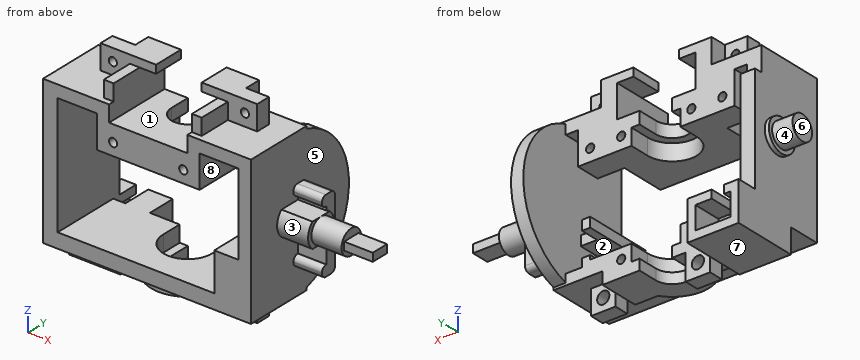
```python
from build123d import *

# Parameters (mm, degrees)
SKETCH_1_R               = 0.5
EXTRUDE_1_DEPTH          = 8.5
SKETCH_2_W               = 3.3
SKETCH_2_H               = 4
SKETCH_2_R               = 0.5
EXTRUDE_2_DEPTH          = 3
EXTRUDE_3_DEPTH          = 3.8
SKETCH_4_W               = 2.8
SKETCH_4_H               = 3
SKETCH_4_R               = 0.5
EXTRUDE_4_DEPTH          = 1.8
SKETCH_5_W               = 1.2
SKETCH_5_H               = 2
EXTRUDE_5_DEPTH          = 4
SKETCH_6_W               = 1.8
SKETCH_6_H               = 15
EXTRUDE_6_DEPTH          = 1
EXTRUDE_7_DEPTH          = 3.5
EXTRUDE_7_DEPTH_BACK     = 4.5
SKETCH_8_W               = 4.3
SKETCH_8_H               = 2
EXTRUDE_8_DEPTH          = 1
EXTRUDE_9_DEPTH          = 1.5
SKETCH_10_R              = 0.75
EXTRUDE_10_DEPTH         = 1.8
SKETCH_12_W              = 3
SKETCH_12_H              = 1.8
EXTRUDE_11_DEPTH         = 3
SKETCH_13_R              = 0.75
CUT_EXTRUDE_1_DEPTH      = 3
SKETCH_14_R              = 0.5
CUT_EXTRUDE_2_DEPTH      = 3
CUT_EXTRUDE_3_DEPTH      = 7
CUT_EXTRUDE_4_DEPTH      = 36.146123542
CUT_EXTRUDE_5_DEPTH      = 12.7
CUT_EXTRUDE_5_DEPTH_BACK = 2
SKETCH_18_W              = 2
SKETCH_18_H              = 1.2
CUT_EXTRUDE_6_DEPTH      = 2.3
EXTRUDE_12_DEPTH         = 1.5
SKETCH_22_R              = 1.5
EXTRUDE_13_DEPTH         = 3
SKETCH_23_R              = 2
EXTRUDE_14_DEPTH         = 0.5
EXTRUDE_START            = 7.5
SKETCH_24_R              = 1.5
EXTRUDE_15_DEPTH         = 7.5
EXTRUDE_16_DEPTH         = 3.5
EXTRUDE_17_DEPTH         = 3.5
EXTRUDE_START_2          = 3.8
EXTRUDE_18_DEPTH         = 3.8


with BuildPart() as part:
    # 草图1 → 凸台-拉伸1 (new body)
    with BuildSketch(Plane(origin=(0, 0, 0), x_dir=(1, 0, 0), z_dir=(0, 1, 0))):
        Polygon((25.5, 0), (25.5, 18), (0, 18), (0, 0), (8.1, 0), (8.1, 2), (17.7, 2), (17.7, 0), align=None)
        with Locations(Location((8.6, 4, 0), (0, 0, 270))):
            Circle(SKETCH_1_R, mode=Mode.SUBTRACT)
        with Locations(Location((17.2, 4, 0), (0, 0, 270))):
            Circle(SKETCH_1_R, mode=Mode.SUBTRACT)
        Polygon((24, 1.5), (19.2, 1.5), (19.2, 5.5), (12.9, 5.5), (6.6, 5.5), (6.6, 1.5), (1.8, 1.5), (1.8, 16.2), (21, 16.2), (21, 11.5), (24, 11.5), align=None, mode=Mode.SUBTRACT)
    extrude(amount=EXTRUDE_1_DEPTH)

    # 草图2 → 凸台-拉伸2 (add)
    # profile 1 of 2: a face of its own
    with BuildSketch(Plane(origin=(0, 8.5, 0), x_dir=(1, 0, 0), z_dir=(0, 1, 0))):
        with Locations((4.95, 3.5)):
            Rectangle(SKETCH_2_W, SKETCH_2_H)
        with Locations(Location((4.8, 4, 0), (0, 0, 270))):
            Circle(SKETCH_2_R, mode=Mode.SUBTRACT)
    # profile 2 of 2: a face of its own
    with BuildSketch(Plane(origin=(0, 8.5, 0), x_dir=(1, 0, 0), z_dir=(0, 1, 0))):
        with Locations((20.85, 3.5)):
            Rectangle(SKETCH_2_W, SKETCH_2_H)
        with Locations(Location((21, 4, 0), (0, 0, 270))):
            Circle(SKETCH_2_R, mode=Mode.SUBTRACT)
    extrude(amount=-EXTRUDE_2_DEPTH)

    # 草图3 → 凸台-拉伸3 (add)
    with BuildSketch(Plane(origin=(0, 8.5, 0), x_dir=(1, 0, 0), z_dir=(0, 1, 0))):
        Polygon((17.7, 0), (17.7, -2), (15.7, -2), (15.7, -3), (17.7, -3), (19.7, -3), (19.7, 0), align=None)
        Polygon((8.1, 0), (6.1, 0), (6.1, -3), (8.1, -3), (10.1, -3), (10.1, -2), (8.1, -2), align=None)
    extrude(amount=-EXTRUDE_3_DEPTH)

    # 草图4 → 凸台-拉伸4 (add)
    # profile 1 of 2: a face of its own
    with BuildSketch(Plane.XZ.offset(-4.7)):
        with Locations((21.1, 1.5)):
            Rectangle(SKETCH_4_W, SKETCH_4_H)
        with Locations(Location((21, 1.5, 0), (0, 0, 270))):
            Circle(SKETCH_4_R, mode=Mode.SUBTRACT)
    # profile 2 of 2: a face of its own
    with BuildSketch(Plane.XZ.offset(-4.7)):
        with Locations((4.7, 1.5)):
            Rectangle(SKETCH_4_W, SKETCH_4_H)
        with Locations(Location((4.8, 1.5, 0), (0, 0, 270))):
            Circle(SKETCH_4_R, mode=Mode.SUBTRACT)
    extrude(amount=-EXTRUDE_4_DEPTH)

    # 草图5 → 凸台-拉伸5 (add)
    with BuildSketch(Plane.XZ.offset(-4.7)):
        with Locations((7.5, 1)):
            Rectangle(SKETCH_5_W, SKETCH_5_H)
        with Locations((18.3, 1)):
            Rectangle(SKETCH_5_W, SKETCH_5_H)
    extrude(amount=EXTRUDE_5_DEPTH)

    # 草图6 → 凸台-拉伸6 (add)
    with BuildSketch(Plane(origin=(0, 8.5, 0), x_dir=(1, 0, 0), z_dir=(0, 1, 0))):
        with Locations((0.9, 10.5)):
            Rectangle(SKETCH_6_W, SKETCH_6_H)
    extrude(amount=EXTRUDE_6_DEPTH)

    # 草图7 → 凸台-拉伸7 (add, two sides: drawn at the far end of the back side and taken through both)
    with BuildSketch(Plane(origin=(0, 8.5, 0), x_dir=(1, 0, 0), z_dir=(0, 1, 0)).offset(-EXTRUDE_7_DEPTH_BACK)):
        Polygon((0, 18), (0, 21), (6.3, 21), (6.3, 16.2), (3.3, 16.2), (3.3, 17.2), (5.3, 17.2), (5.3, 20), (1, 20), (1, 17.2), (1.8, 17.2), (1.8, 16.2), (0, 16.2), align=None)
    extrude(amount=EXTRUDE_7_DEPTH + EXTRUDE_7_DEPTH_BACK)

    # 草图8 → 凸台-拉伸8 (add)
    with BuildSketch(Plane.XZ.offset(-4)):
        with Locations((3.15, -19)):
            Rectangle(SKETCH_8_W, SKETCH_8_H)
    extrude(amount=-EXTRUDE_8_DEPTH)

    # 草图9 → 凸台-拉伸9 (add)
    with BuildSketch(Plane(origin=(0, 0, -18), x_dir=(-1, 0, 0), z_dir=(0, 0, -1))):
        with BuildLine():
            Line((-10.95, 8.5), (-10.95, 6))
            ThreePointArc((-10.95, 6), (-12.95, 4), (-14.95, 6))
            Line((-14.95, 6), (-14.95, 8.5))
            Line((-14.95, 8.5), (-19.5, 8.5))
            Line((-19.5, 8.5), (-19.5, 3.5))
            Line((-19.5, 3.5), (-16.691657387, 3.5))
            ThreePointArc((-16.691657387, 3.5), (-12.95, 1.5), (-9.208342613, 3.5))
            Line((-9.208342613, 3.5), (-6.3, 3.5))
            Line((-6.3, 3.5), (-6.3, 8.5))
            Line((-6.3, 8.5), (-10.95, 8.5))
        make_face()
    extrude(amount=EXTRUDE_9_DEPTH)

    # 草图10 → 凸台-拉伸10 (add)
    with BuildSketch(Plane(origin=(0, 8.5, 0), x_dir=(1, 0, 0), z_dir=(0, 1, 0))):
        Polygon((6.3, 22.7), (6.3, 19.5), (9.3, 19.5), (9.3, 21.1), (9.3, 22.7), align=None)
        with Locations(Location((7.8, 21.1, 0), (0, 0, 270))):
            Circle(SKETCH_10_R, mode=Mode.SUBTRACT)
    extrude(amount=-EXTRUDE_10_DEPTH)

    # 草图12 → 凸台-拉伸11 (add)
    with BuildSketch(Plane(origin=(0, 0, -18), x_dir=(-1, 0, 0), z_dir=(0, 0, -1))):
        with Locations((-21, 5.6)):
            Rectangle(SKETCH_12_W, SKETCH_12_H)
    extrude(amount=EXTRUDE_11_DEPTH)

    # 草图13 → 切除-拉伸1 (cut)
    with BuildSketch(Plane(origin=(0, 6.5, 0), x_dir=(1, 0, 0), z_dir=(0, 1, 0))):
        with Locations(Location((21, 19.5, 0), (0, 0, 270))):
            Circle(SKETCH_13_R)
    extrude(amount=-CUT_EXTRUDE_1_DEPTH, mode=Mode.SUBTRACT)

    # 草图14 → 切除-拉伸2 (cut)
    with BuildSketch(Plane(origin=(0, 8.5, 0), x_dir=(1, 0, 0), z_dir=(0, 1, 0))):
        with Locations(Location((17.2, 17.5, 0), (0, 0, 270))):
            Circle(SKETCH_14_R)
        with Locations(Location((8.6, 17.5, 0), (0, 0, 270))):
            Circle(SKETCH_14_R)
    extrude(amount=-CUT_EXTRUDE_2_DEPTH, mode=Mode.SUBTRACT)

    # 草图15 → 切除-拉伸3 (cut)
    with BuildSketch(Plane(origin=(0, 8.5, 0), x_dir=(1, 0, 0), z_dir=(0, 1, 0))):
        Polygon((21, 15.7), (21, 12.7), (24, 12.7), (24, 16.7), (22, 16.7), (22, 15.7), align=None)
    extrude(amount=-CUT_EXTRUDE_3_DEPTH, mode=Mode.SUBTRACT)

    # 草图16 → 切除-拉伸4 (cut, through all)
    with BuildSketch(Plane(origin=(0, 0, -18), x_dir=(-1, 0, 0), z_dir=(0, 0, -1))):
        with BuildLine():
            Line((-14.95, 8.5), (-10.95, 8.5))
            Line((-10.95, 8.5), (-10.95, 6))
            ThreePointArc((-10.95, 6), (-12.95, 4), (-14.95, 6))
            Line((-14.95, 6), (-14.95, 8.5))
        make_face()
    extrude(amount=-CUT_EXTRUDE_4_DEPTH, mode=Mode.SUBTRACT)

    # 草图17 → 切除-拉伸5 (cut, two sides: drawn at the far end of the back side and taken through both)
    with BuildSketch(Plane.XY.offset(-16.2).offset(-CUT_EXTRUDE_5_DEPTH_BACK)):
        with BuildLine():
            Line((15.95, 6), (15.95, 8.5))
            Line((15.95, 8.5), (9.95, 8.5))
            Line((9.95, 8.5), (9.95, 6))
            ThreePointArc((9.95, 6), (12.95, 3), (15.95, 6))
        make_face()
    extrude(amount=CUT_EXTRUDE_5_DEPTH + CUT_EXTRUDE_5_DEPTH_BACK, mode=Mode.SUBTRACT)

    # 草图18 → 切除-拉伸6 (cut)
    with BuildSketch(Plane(origin=(0, 8.5, 0), x_dir=(1, 0, 0), z_dir=(0, 1, 0))):
        with Locations((23, 12.1)):
            Rectangle(SKETCH_18_W, SKETCH_18_H)
    extrude(amount=-CUT_EXTRUDE_6_DEPTH, mode=Mode.SUBTRACT)

    # 草图19 → 凸台-拉伸12 (add)
    with BuildSketch(Plane(origin=(25.5, 0, 0), x_dir=(0, 0, -1), z_dir=(1, 0, 0))):
        with BuildLine():
            Line((0.30001254, 8.5), (17.69998746, 8.5))
            ThreePointArc((17.69998746, 8.5), (9, 14.998364198), (0.30001254, 8.5))
        make_face()
    extrude(amount=-EXTRUDE_12_DEPTH)

    # 草图22 → 凸台-拉伸13 (add)
    with BuildSketch(Plane.ZY):
        with Locations(Location((-9, 6, 0), (0, 0, 180))):
            Circle(SKETCH_22_R)
    extrude(amount=EXTRUDE_13_DEPTH)

    # 草图23 → 凸台-拉伸14 (add)
    with BuildSketch(Plane.ZY):
        with Locations(Location((-9, 6, 0), (0, 0, 180))):
            Circle(SKETCH_23_R)
    extrude(amount=EXTRUDE_14_DEPTH)

    # 草图24 → 凸台-拉伸15 (add)
    with BuildSketch(Plane(origin=(25.5, 0, 0), x_dir=(0, 0, -1), z_dir=(1, 0, 0)).offset(EXTRUDE_START)):
        with Locations(Location((9, 6, 0), (0, 0, 180))):
            Circle(SKETCH_24_R)
    extrude(amount=-EXTRUDE_15_DEPTH)

    # 草图25 → 凸台-拉伸16 (add)
    with BuildSketch(Plane(origin=(33, 0, 0), x_dir=(0, 0, -1), z_dir=(1, 0, 0))):
        Polygon((9.5, 6), (9.5, 7.090871211), (8.5, 7.090871211), (8.5, 4.909128789), (9.5, 4.909128789), align=None)
    extrude(amount=EXTRUDE_16_DEPTH)

    # 草图26 → 凸台-拉伸17 (add)
    with BuildSketch(Plane(origin=(25.5, 0, 0), x_dir=(0, 0, -1), z_dir=(1, 0, 0))):
        with BuildLine():
            Line((9, 8.498364198), (6.3, 8.498364198))
            ThreePointArc((6.3, 8.498364198), (5.875735931, 8.322628267), (5.7, 7.898364198))
            Line((5.7, 7.898364198), (5.7, 7.098364198))
            ThreePointArc((5.7, 7.098364198), (5.875735931, 6.674100129), (6.3, 6.498364198))
            Line((6.3, 6.498364198), (6.4, 6.498364198))
            ThreePointArc((6.4, 6.498364198), (6.824264069, 6.674100129), (7, 7.098364198))
            Line((7, 7.098364198), (7, 7.198364198))
            Line((7, 7.198364198), (13.4, 7.198364198))
            Line((13.4, 7.198364198), (13.4, 7.098364198))
            ThreePointArc((13.4, 7.098364198), (13.575735931, 6.674100129), (14, 6.498364198))
            Line((14, 6.498364198), (14.1, 6.498364198))
            ThreePointArc((14.1, 6.498364198), (14.524264069, 6.674100129), (14.7, 7.098364198))
            Line((14.7, 7.098364198), (14.7, 7.898364198))
            ThreePointArc((14.7, 7.898364198), (14.524264069, 8.322628267), (14.1, 8.498364198))
            Line((14.1, 8.498364198), (9, 8.498364198))
        make_face()
    extrude(amount=EXTRUDE_17_DEPTH)

    # 草图27 → 凸台-拉伸18 (add)
    with BuildSketch(Plane(origin=(25.5, 0, 0), x_dir=(0, 0, -1), z_dir=(1, 0, 0)).offset(EXTRUDE_START_2)):
        with BuildLine():
            Line((7.5, 6), (7.5, 7.322875656))
            ThreePointArc((7.5, 7.322875656), (9, 8), (10.5, 7.322875656))
            Line((10.5, 7.322875656), (10.5, 4.677124344))
            ThreePointArc((10.5, 4.677124344), (9, 4), (7.5, 4.677124344))
            Line((7.5, 4.677124344), (7.5, 6))
        make_face()
    extrude(amount=-EXTRUDE_18_DEPTH)


solid = part.part
```
Input: part model. Units: mm. Frame: model coordinates. Face numbers are marked on the shaded views. A direction names the side the tool comes from. Coordinates: 2 decimals unless noted, no trailing zeros. Write each loop counter-clockwise with the first axis right and the second up, starting at its lowest first coordinate (ties: lowest second). Pieces come first, ordered by that corner, then holes. Notation, with made-up numbers: (52.5, 79) -> (81.5, 79) arc R19 ccw to (81.5, 112) -> close; hole circle Ø5 at (-9, 66). An arc over 180 degrees is marked (long way). Answer as a JSON object with one key per item and string values.
1. Access query for the marked faces 1, 2, 3, 4 and 5. Directions: +Z, -Z, +X, -X, +Y, -Y. A direction counts if a zero-diameter tool reaches every point of the face in a straight line with its end or side. Return the directions, or none.
Result set:
{"face 1": "+Y, -Y", "face 2": "+Y", "face 3": "+X, -Y", "face 4": "-X", "face 5": "+X"}
2. First-contact query: P1, Ø6, axis at x = 31, y = 3, coming from the -Z side; P2, Ø0.9, axis at y = 5.5, z = 1.5, coming from the +X side; P3, Ø5, axis at x = 1.5, y = 7, coming from the -Z side. Flat tips, straight axial feed; report the tip coordinate or a pass-through.
Result set:
{"P1": "stops at z = -10.5", "P2": "stops at x = 22.5", "P3": "stops at z = -21"}
3. Section B-B on x = 12.95. Return the cut outline in (y, z).
Result set:
{"outline": "(0, -18) -> (1.5, -18) -> (1.5, -19.5) -> (4, -19.5) -> (4, -18.2) -> (3, -18.2) -> (3, -16.2) -> (0, -16.2) -> close; (0, -5.5) -> (3, -5.5) -> (3, -3.5) -> (4, -3.5) -> (4, -2) -> (0, -2) -> close"}
4. Material intervals for line 1 (X direction, y = 6.6, z = -17.5); line 2 (X direction, y = 7.4, z = -21.1); line 3 (X direction, y = 9, z = -11), sorted ascending. Write a range as from..to.
Result set:
{"line 1": "x = 0..8.1, 9.1..9.95, 15.95..16.7, 17.7..25.5", "line 2": "x = 6.3..7.05, 8.55..9.3", "line 3": "x = 0..1.8, 24..25.5"}
5. Section A-A on z = 1.5. Return the cut outline in (x, y), then the cut area to 3 significant figures.
Result set:
{"outline": "(3.3, 4.7) -> (4.3, 4.7) -> (4.3, 6.5) -> (3.3, 6.5) -> close; (5.3, 4.7) -> (6.9, 4.7) -> (6.9, 0.7) -> (8.1, 0.7) -> (8.1, 8.5) -> (6.1, 8.5) -> (6.1, 6.5) -> (5.3, 6.5) -> close; (17.7, 0.7) -> (18.9, 0.7) -> (18.9, 4.7) -> (20.5, 4.7) -> (20.5, 6.5) -> (19.7, 6.5) -> (19.7, 8.5) -> (17.7, 8.5) -> close; (21.5, 4.7) -> (22.5, 4.7) -> (22.5, 6.5) -> (21.5, 6.5) -> close", "area": "31.3 mm2"}
6. Section D-D on y = 10.25. Return the cut outline in (x, z).
Result set:
{"outline": "(0, -21) -> (6.3, -21) -> (6.3, -16.2) -> (3.3, -16.2) -> (3.3, -17.2) -> (5.3, -17.2) -> (5.3, -20) -> (1, -20) -> (1, -17.2) -> (1.8, -17.2) -> (1.8, -16.2) -> (0, -16.2) -> close; (24, -16.98) -> (25.5, -16.98) -> (25.5, -1.02) -> (24, -1.02) -> close"}
7. Mould query, pull axis X, two halves, no side actions, for the marked faces 6, 7 and 8. Classes: released by +X, released by -X, zero draft, split by the parting line, or undercut.
Result set:
{"face 6": "released by -X", "face 7": "zero draft", "face 8": "undercut"}
8. Section C-C on x = 4.8. Count the separate pieces of the cut face and the enclosed holes in it, then the cut area to 4 significant figures.
Result set:
{"separate pieces": "4", "enclosed holes": "0", "area": "54.15 mm2"}
